```python
from build123d import *

# Parameters (mm, degrees)
PAD_DEPTH              = 13.4
CYLINDER_W             = 6.7
CYLINDER_H             = 298.45
CYLINDER_ANGLE         = 180
CYLINDER001_R          = 99.483333
CYLINDER001_DEPTH      = 32
BOX_W                  = 149.225
BOX_H                  = 30
BOX_DEPTH              = 21
BOX001_W               = 33
BOX001_H               = 149.225
BOX001_DEPTH           = 22
CYLINDER002_R          = 3.7
CYLINDER002_DEPTH      = 105
LINEARPATTERN_COUNT    = 3
LINEARPATTERN_PITCH    = 74.6125
CYLINDER003_R          = 1.85
CYLINDER003_DEPTH      = 100
LINEARPATTERN001_COUNT = 3
LINEARPATTERN001_PITCH = 74.6125


with BuildPart() as part:
    # Sketch → Pad (new body)
    with BuildSketch(Plane.XY):
        Polygon((0, 0), (298.45, 0), (0, 298.45), align=None)
    extrude(amount=PAD_DEPTH)

    # Cylinder → Cylinder (revolve, cut)
    with BuildSketch(Plane(origin=(0, 0, 6.7), x_dir=(0, 0, 1), z_dir=(-1, 0, 0))):
        with Locations((3.35, 149.225)):
            Rectangle(CYLINDER_W, CYLINDER_H)
    revolve(axis=Axis((0, 0, 6.7), (0, 1, 0)), revolution_arc=CYLINDER_ANGLE, mode=Mode.SUBTRACT)

    # Cylinder001 → Cylinder001 (cut)
    with BuildSketch(Plane(origin=(149.225, 149.225, -8), x_dir=(1, 0, 0), z_dir=(0, 0, 1))):
        Circle(CYLINDER001_R)
    extrude(amount=CYLINDER001_DEPTH, mode=Mode.SUBTRACT)

    # Box → Box (cut)
    with BuildSketch(Plane(origin=(149.225, 79.741667, 17), x_dir=(1, 0, 0), z_dir=(0, 0, -1))):
        with Locations((74.6125, 15)):
            Rectangle(BOX_W, BOX_H)
    extrude(amount=BOX_DEPTH, mode=Mode.SUBTRACT)

    # Box001 → Box001 (cut)
    with BuildSketch(Plane(origin=(49.741667, 303.579167, 17), x_dir=(1, 0, 0), z_dir=(0, 0, -1))):
        with Locations((16.5, 74.6125)):
            Rectangle(BOX001_W, BOX001_H)
    extrude(amount=BOX001_DEPTH, mode=Mode.SUBTRACT)

    # Cylinder002 → Cylinder002 (cut)
    with BuildSketch(Plane(origin=(74.6125, 5, 6.7), x_dir=(-1, 0, 0), z_dir=(0, 1, 0))):
        Circle(CYLINDER002_R)
    cylinder002 = extrude(amount=CYLINDER002_DEPTH, mode=Mode.SUBTRACT)

    # LinearPattern: Cylinder002 ×3
    with Locations(*[(i * LINEARPATTERN_PITCH, 0, 0) for i in range(1, LINEARPATTERN_COUNT)]):
        add(cylinder002, mode=Mode.SUBTRACT)

    # Cylinder003 → Cylinder003 (cut)
    with BuildSketch(Plane(origin=(74.6125, 0, 6.7), x_dir=(-1, 0, 0), z_dir=(0, 1, 0))):
        Circle(CYLINDER003_R)
    cylinder003 = extrude(amount=CYLINDER003_DEPTH, mode=Mode.SUBTRACT)

    # LinearPattern001: Cylinder003 ×3
    with Locations(*[(i * LINEARPATTERN001_PITCH, 0, 0) for i in range(1, LINEARPATTERN001_COUNT)]):
        add(cylinder003, mode=Mode.SUBTRACT)


solid = part.part
```
Input: part model. Units: mm. Frame: model coordinates. A direction names the side the tool comes from. Give positions to 0.01 mm unless a question says otherwise; leave off trailing zeros. Order: outer loops, then holes, each group sorted by start corner. A loop starts at its lowest first (then second) coordinate and runs counter-clockwise, first axis right, second up. Notation, with made-up numbers: (-6, 13.5) - (33, 13.5) arc R19 cw to (33, 49.5) - close; hole circle Ø6 at (33.25, 39). An arc over 180 degrees is marked (long way). Put each result on its own line as item: value.
Item 1: Access query for faces 4 (the flat face through (60, 84, 0)), 5 (the flat face through (49.742, 202, 7)), 6 (the flat face through (151, 5, 8)). Directions: +Z, -Z, +X, -X, +Y, -Y. A direction counts if a zero-diameter tool reaches every point of the face in a straight line with its end or side. Return the directions, or none.
Found:
face 4: -Z, +X, -X, +Y, -Y
face 5: +Z, -Z, +X, +Y
face 6: +Y
Item 2: Contact query for flat-ended pins moving along their axis: pin 1 (6 mm diameter, centred on x = 149.225, z = 6.7, fed in from +Y); pin 2 (3 mm diameter, centred on y = 111.5, z = 11, fed in from -X); pin 3 (6 mm diameter, centred on x = 159, z = 7, fed in from +Y). Output: stop coordinate, or through.
Found:
pin 1: stops at y = 5
pin 2: stops at x = 3.35
pin 3: stops at y = 49.74
Item 3: Ray query, L1, parallel to X at y = 1.95, z = 6.7 (1 decimal); L2, parallel to X at y = 2.15, z = 6.7 (1 decimal); L3, parallel to X at y = 248.5, z = 11.25. Return the intervals inside material, ascending. Write a range as from..to.
Found:
L1: x = 6.7..72.8, 76.5..147.4, 151.1..222, 225.7..296.5
L2: x = 6.7..72.8, 76.5..147.4, 151.1..222, 225.7..296.3
L3: x = 4.92..49.74
Item 4: Draft query along X for faces 1 (the flat face through (60, 84, 13.4)), 2 (the flat face through (25.22, 273.23, 6.61)), 3 (the cylindrical face through (227.534, 27.058, 6.863)). Return one class per face: +X half, -X half, draft (parallel to the pull), parting line (faces both ways), or undercut.
Found:
face 1: draft
face 2: +X half
face 3: undercut
Item 5: Section query B-B, the plane y = 221. Return loops of the section in (x, z).
Found:
outline: (0, 0) - (49.74, 0) - (49.74, 13.4) - (0, 13.4) arc R6.7 cw to start
Item 6: Section query A-A, the plane x = 209. Return loops of the section in (y, z), then the cut area to 3 significant figures.
Found:
outline: (0, 0) - (49.74, 0) - (49.74, 13.4) - (0, 13.4) - close
area: 667 mm^2
